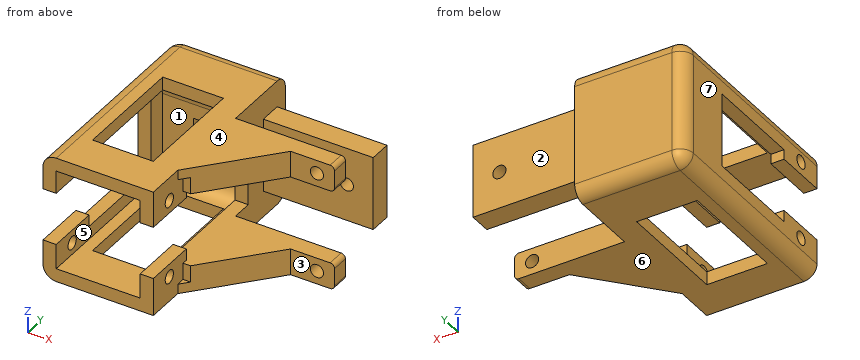
```python
from build123d import *

# Parameters (mm, degrees)
SKETCH4_W            = 25.1
SKETCH4_H            = 28.75
BOSS_EXTRUDE2_DEPTH  = 53
SKETCH5_W            = 19.1
SKETCH5_H            = 22.75
CUT_EXTRUDE1_DEPTH   = 21.67
FILLET1_R            = 4.1
SKETCH6_W            = 5
SKETCH6_H            = 8
CUT_EXTRUDE2_DEPTH   = 4.67
SKETCH7_W            = 16.769550268
SKETCH7_H            = 35.14
CUT_EXTRUDE3_DEPTH   = 40
SKETCH8_W            = 13.798322684
SKETCH8_H            = 35.14
CUT_EXTRUDE4_DEPTH   = 40
BOSS_EXTRUDE3_DEPTH  = 17
SKETCH10_W           = 3
SKETCH10_H           = 9
BOSS_EXTRUDE4_DEPTH  = 13.8
SKETCH11_W           = 3
SKETCH11_H           = 9
BOSS_EXTRUDE5_DEPTH  = 13.8
SKETCH12_W           = 3
SKETCH12_H           = 12
BOSS_EXTRUDE6_DEPTH  = 16.77
SKETCH24_R           = 1.5
CUT_EXTRUDE6_DEPTH   = 40.8
SKETCH25_W           = 28.75
SKETCH25_H           = 21.925089144
CUT_EXTRUDE7_DEPTH   = 40.8
SKETCH26_W           = 11.913987102
SKETCH26_H           = 12
CUT_EXTRUDE8_DEPTH   = 40.8
SKETCH30_W           = 28.75
SKETCH30_H           = 8.02
BOSS_EXTRUDE10_DEPTH = 30
SKETCH32_W           = 5.990224866
SKETCH32_H           = 21.060252184
BOSS_EXTRUDE13_DEPTH = 30
CUT_EXTRUDE9_DEPTH   = 30
SKETCH36_W           = 5
SKETCH36_H           = 28.75
CUT_EXTRUDE10_DEPTH  = 30
SKETCH38_W           = 5.99
SKETCH38_H           = 8.02
CUT_EXTRUDE11_DEPTH  = 25
SKETCH39_R           = 1.5
CUT_EXTRUDE12_DEPTH  = 25
SKETCH40_R           = 1.5
CUT_EXTRUDE13_DEPTH  = 25
FILLET4_R            = 3
FILLET5_R            = 3
FILLET7_R            = 1
SKETCH41_W           = 16.77
SKETCH41_H           = 3
CUT_EXTRUDE14_DEPTH  = 25
CUT_EXTRUDE15_DEPTH  = 3.79
CUT_EXTRUDE16_DEPTH  = 3.79


with BuildPart() as part:
    # Sketch4 → Boss-Extrude2 (new body)
    with BuildSketch(Plane(origin=(0, 0, 0), x_dir=(1, 0, 0), z_dir=(0, 1, 0))):
        Rectangle(SKETCH4_W, SKETCH4_H)
    extrude(amount=BOSS_EXTRUDE2_DEPTH)

    # Sketch5 → Cut-Extrude1 (cut)
    with BuildSketch(Plane(origin=(0, 0, 0), x_dir=(-1, 0, 0), z_dir=(0, -1, 0))):
        Rectangle(SKETCH5_W, SKETCH5_H)
    extrude(amount=-CUT_EXTRUDE1_DEPTH, mode=Mode.SUBTRACT)

    # Fillet1
    fillet1_edges = [part.edges().sort_by_distance(p)[0] for p in [
        (0, 21.67, -11.375),
        (0, 21.67, 11.375),
    ]]
    fillet(fillet1_edges, radius=FILLET1_R)

    # Sketch6 → Cut-Extrude2 (cut)
    with BuildSketch(Plane(origin=(0, 21.67, 0), x_dir=(-1, 0, 0), z_dir=(0, -1, 0))):
        Rectangle(SKETCH6_W, SKETCH6_H)
    extrude(amount=-CUT_EXTRUDE2_DEPTH, mode=Mode.SUBTRACT)

    # Sketch7 → Cut-Extrude3 (cut)
    with BuildSketch(Plane(origin=(12.55, 0, 0), x_dir=(0, 0, -1), z_dir=(1, 0, 0))):
        Rectangle(SKETCH7_W, SKETCH7_H)
    extrude(amount=-CUT_EXTRUDE3_DEPTH, mode=Mode.SUBTRACT)

    # Sketch8 → Cut-Extrude4 (cut)
    with BuildSketch(Plane(origin=(0, 0, -14.375), x_dir=(-1, 0, 0), z_dir=(0, 0, -1))):
        Rectangle(SKETCH8_W, SKETCH8_H)
    extrude(amount=-CUT_EXTRUDE4_DEPTH, mode=Mode.SUBTRACT)

    # Sketch9 → Boss-Extrude3 (add)
    with BuildSketch(Plane.XZ):
        Polygon((-9.55, 8.384775134), (-12.55, 8.384775134), (-12.55, 14.375), (-6.899161342, 14.375), (-6.899161342, 11.375), (-9.55, 11.375), align=None)
        Polygon((-9.55, -8.384775134), (-12.55, -8.384775134), (-12.55, -14.375), (-6.899161342, -14.375), (-6.899161342, -11.375), (-9.55, -11.375), align=None)
        Polygon((6.899161342, -11.375), (6.899161342, -14.375), (12.55, -14.375), (12.55, -8.384775134), (9.55, -8.384775134), (9.55, -11.375), align=None)
        Polygon((9.55, 8.384775134), (12.55, 8.384775134), (12.55, 14.375), (6.899161342, 14.375), (6.899161342, 11.375), (9.55, 11.375), align=None)
    extrude(amount=BOSS_EXTRUDE3_DEPTH)

    # Sketch10 → Boss-Extrude4 (add)
    with BuildSketch(Plane(origin=(-6.899161342, 0, 0), x_dir=(0, 0, -1), z_dir=(1, 0, 0))):
        with Locations((-12.875, -12.5)):
            Rectangle(SKETCH10_W, SKETCH10_H)
    extrude(amount=BOSS_EXTRUDE4_DEPTH)

    # Sketch11 → Boss-Extrude5 (add)
    with BuildSketch(Plane.ZY.offset(-6.899161342)):
        with Locations((-12.875, -12.5)):
            Rectangle(SKETCH11_W, SKETCH11_H)
    extrude(amount=BOSS_EXTRUDE5_DEPTH)

    # Sketch12 → Boss-Extrude6 (add)
    with BuildSketch(Plane.XY.offset(-8.384775134)):
        with Locations((-11.05, -11)):
            Rectangle(SKETCH12_W, SKETCH12_H)
        with Locations((11.05, -11)):
            Rectangle(SKETCH12_W, SKETCH12_H)
    extrude(amount=BOSS_EXTRUDE6_DEPTH)

    # Sketch24 → Cut-Extrude6 (cut)
    with BuildSketch(Plane(origin=(12.55, 0, 0), x_dir=(0, 0, -1), z_dir=(1, 0, 0))):
        with Locations((8.675, -11.18)):
            Circle(SKETCH24_R)
        with Locations((-9.075, -11.18)):
            Circle(SKETCH24_R)
    extrude(amount=-CUT_EXTRUDE6_DEPTH, mode=Mode.SUBTRACT)

    # Sketch25 → Cut-Extrude7 (cut)
    with BuildSketch(Plane.ZY.offset(12.55)):
        with Locations((0, 42.037455428)):
            Rectangle(SKETCH25_W, SKETCH25_H)
    extrude(amount=-CUT_EXTRUDE7_DEPTH, mode=Mode.SUBTRACT)

    # Sketch26 → Cut-Extrude8 (cut)
    with BuildSketch(Plane.ZY.offset(12.55)):
        with Locations((0.21531302, -11)):
            Rectangle(SKETCH26_W, SKETCH26_H)
    extrude(amount=-CUT_EXTRUDE8_DEPTH, mode=Mode.SUBTRACT)

    # Sketch30 → Boss-Extrude10 (add)
    with BuildSketch(Plane(origin=(12.55, 0, 0), x_dir=(0, 0, -1), z_dir=(1, 0, 0))):
        with Locations((0, 27.064910856)):
            Rectangle(SKETCH30_W, SKETCH30_H)
    extrude(amount=BOSS_EXTRUDE10_DEPTH)

    # Sketch32 → Boss-Extrude13 (add)
    with BuildSketch(Plane(origin=(12.55, 0, 0), x_dir=(0, 0, -1), z_dir=(1, 0, 0))):
        with Locations((-11.379887567, 2.424784764)):
            Rectangle(SKETCH32_W, SKETCH32_H)
        with Locations((11.379887567, 2.424784764)):
            Rectangle(SKETCH32_W, SKETCH32_H)
    extrude(amount=BOSS_EXTRUDE13_DEPTH)

    # Sketch35 → Cut-Extrude9 (cut)
    with BuildSketch(Plane(origin=(0, 0, -14.375), x_dir=(-1, 0, 0), z_dir=(0, 0, -1))):
        Polygon((-42.55, 8.954910856), (-27.55, 8.954910856), (-12.55, -8.105341328), (-42.55, -8.105341328), align=None)
    extrude(amount=-CUT_EXTRUDE9_DEPTH, mode=Mode.SUBTRACT)

    # Sketch36 → Cut-Extrude10 (cut)
    with BuildSketch(Plane(origin=(0, 31.074910856, 0), x_dir=(1, 0, 0), z_dir=(0, 1, 0))):
        with Locations((40.05, 0)):
            Rectangle(SKETCH36_W, SKETCH36_H)
    extrude(amount=-CUT_EXTRUDE10_DEPTH, mode=Mode.SUBTRACT)

    # Sketch38 → Cut-Extrude11 (cut)
    with BuildSketch(Plane(origin=(37.55, 0, 0), x_dir=(0, 0, -1), z_dir=(1, 0, 0))):
        with Locations((-11.38, 27.064910856)):
            Rectangle(SKETCH38_W, SKETCH38_H)
        with Locations((11.38, 27.064910856)):
            Rectangle(SKETCH38_W, SKETCH38_H)
    extrude(amount=-CUT_EXTRUDE11_DEPTH, mode=Mode.SUBTRACT)

    # Sketch39 → Cut-Extrude12 (cut)
    with BuildSketch(Plane(origin=(0, 8.954910856, 0), x_dir=(-1, 0, 0), z_dir=(0, -1, 0))):
        with Locations(Location((-33.55, 11.379887567, 0), (0, 0, 90))):
            Circle(SKETCH39_R)
        with Locations(Location((-33.55, -11.379887567, 0), (0, 0, 90))):
            Circle(SKETCH39_R)
    extrude(amount=-CUT_EXTRUDE12_DEPTH, mode=Mode.SUBTRACT)

    # Sketch40 → Cut-Extrude13 (cut)
    with BuildSketch(Plane.XZ.offset(-23.054910856)):
        with Locations(Location((31.55, 0, 0), (0, 0, 270))):
            Circle(SKETCH40_R)
    extrude(amount=-CUT_EXTRUDE13_DEPTH, mode=Mode.SUBTRACT)

    # Fillet4
    fillet4_edges = [part.edges().sort_by_distance(p)[0] for p in [
        (-12.55, 31.074910856, 0),
        (0, 31.074910856, 14.375),
        (0, 31.074910856, -14.375),
    ]]
    fillet(fillet4_edges, radius=FILLET4_R)

    # Fillet5
    # the kernel refuses this fillet: 3 mm, written as the material it takes off along each edge
    with BuildSketch(Plane(origin=(-9.55, 28.074910856, 11.375), x_dir=(0, 0, 1), z_dir=(-1, 0, 0))) as fillet5_piece_1_section:
        Polygon((0, 0), (FILLET5_R, 0), (FILLET5_R, FILLET5_R), (0, FILLET5_R), align=None)
    fillet5_piece_1 = extrude(amount=FILLET5_R, mode=Mode.PRIVATE)
    fillet5_piece_1 = fillet5_piece_1 - Plane(origin=(-9.55, 28.074910856, 11.375), x_dir=(0, -0.7071067811865475, -0.7071067811865475), z_dir=(-1, 0, 0)) * Sphere(FILLET5_R, mode=Mode.PRIVATE)
    add(fillet5_piece_1, mode=Mode.SUBTRACT)
    with BuildSketch(Plane(origin=(-9.55, 28.074910856, -11.375), x_dir=(-1, 0, 0), z_dir=(0, 0, -1))) as fillet5_piece_2_section:
        Polygon((0, 0), (FILLET5_R, 0), (FILLET5_R, FILLET5_R), (0, FILLET5_R), align=None)
    fillet5_piece_2 = extrude(amount=FILLET5_R, mode=Mode.PRIVATE)
    fillet5_piece_2 = fillet5_piece_2 - Plane(origin=(-9.55, 28.074910856, -11.375), x_dir=(0.7071067811865475, -0.7071067811865475, 0), z_dir=(0, 0, -1)) * Sphere(FILLET5_R, mode=Mode.PRIVATE)
    add(fillet5_piece_2, mode=Mode.SUBTRACT)
    with BuildSketch(Plane(origin=(-12.55, 28.074910856, -14.375), x_dir=(1, 0, 0), z_dir=(0, -1, 0))) as fillet5_piece_3:
        with BuildLine():
            CenterArc((FILLET5_R, FILLET5_R), FILLET5_R, 180, 90)
            Line((0, FILLET5_R), (0, 0))
            Line((0, 0), (FILLET5_R, 0))
        make_face()
    extrude(amount=52.574910856, mode=Mode.SUBTRACT)
    with BuildSketch(Plane(origin=(-12.55, -24.5, 14.375), x_dir=(0, 0, -1), z_dir=(0, 1, 0))) as fillet5_piece_4:
        with BuildLine():
            CenterArc((FILLET5_R, -FILLET5_R), FILLET5_R, 90, 90)
            Line((0, -FILLET5_R), (0, 0))
            Line((0, 0), (FILLET5_R, 0))
        make_face()
    extrude(amount=52.574910856, mode=Mode.SUBTRACT)

    # Fillet7
    fillet7_edges = [part.edges().sort_by_distance(p)[0] for p in [
        (37.55, 10.954910856, -14.375),
        (37.55, 10.954910856, -8.384775134),
        (37.55, 10.954910856, 14.375),
        (37.55, 10.954910856, 8.384775134),
    ]]
    fillet(fillet7_edges, radius=FILLET7_R)

    # Sketch41 → Cut-Extrude14 (cut)
    with BuildSketch(Plane(origin=(37.55, 0, 0), x_dir=(0, 0, -1), z_dir=(1, 0, 0))):
        with Locations((0, 29.574910856)):
            Rectangle(SKETCH41_W, SKETCH41_H)
    extrude(amount=-CUT_EXTRUDE14_DEPTH, mode=Mode.SUBTRACT)

    # Sketch43 → Cut-Extrude15 (cut)
    with BuildSketch(Plane(origin=(0, 0, 8.384775134), x_dir=(-1, 0, 0), z_dir=(0, 0, -1))):
        Polygon((-12.55, -8.105341328), (-12.55, -6.175341328), (-14.24692685, -6.175341328), align=None)
    extrude(amount=-CUT_EXTRUDE15_DEPTH, mode=Mode.SUBTRACT)

    # Sketch44 → Cut-Extrude16 (cut)
    with BuildSketch(Plane.XY.offset(-8.384775134)):
        Polygon((12.55, -8.105341328), (12.55, -6.175341328), (14.24692685, -6.175341328), align=None)
    extrude(amount=-CUT_EXTRUDE16_DEPTH, mode=Mode.SUBTRACT)


solid = part.part
```
Can you work these out from the model? Positions are in its coordinate system, mm. Face numbers are marked on the shaded views. A direction names the side the tool comes from. Give positions to 0.01 mm unless a question says otherwise; leave off trailing zeros. Order: outer loops, then holes, each group sorted by start corner. A loop starts at its lowest first (then second) coordinate and runs counter-clockwise, first axis right, second up. Notation, with made-up numbers: M 62,52 L 111,52 A12 cw 111,73 Z; hole C 81.5,-1 d7. An arc over 180 degrees is marked long. One line per item, written item: value.
1) I want a section at C-C, the plane z = 0. List the corners of the cut face in (x, y) for me, plus the area to 3 significant figures.
Answer sheet:
outline: M -12.55,17.57 L -9.55,17.57 L -9.55,21.67 L -2.5,21.67 L -2.5,26.34 L 2.5,26.34 L 2.5,21.67 L 9.55,21.67 L 9.55,17.57 L 12.55,17.57 L 12.55,23.05 L 30.05,23.05 L 30.05,28.07 L 12.55,28.07 L 12.55,31.07 L -9.55,31.07 A3 ccw -12.55,28.07 Z; M 33.05,23.05 L 37.55,23.05 L 37.55,28.07 L 33.05,28.07 Z
area: 346 mm^2
2) For P1, Ø3, axis at x = 18.5, z = -4, coming from the +Y side; P2, Ø7.5, axis at x = 4.5, z = 2, coming from the -Y side; P3, Ø2.5, axis at y = 0.5, z = -13.5, coming from the +X side, each with a flat end and sliding along its axis, tell me the tip position at first contact or that it passes through.
Answer sheet:
P1: stops at y = 28.07
P2: stops at y = 21.67
P3: stops at x = 21.22
3) We'd pull the mould along Z, two halves only. Please class the marked faces 5, 6 and 7: released by +Z, released by -Z, zero draft, split by the parting line, or undercut.
Answer sheet:
face 5: undercut
face 6: released by -Z
face 7: zero draft
4) Please list where these lines run through material, in increasing order: line 1 along Z through (x, y) = (-8.5, 14.5) (3 decimals); line 2 along X through (y, z) = (17, -9.25); line 3 along Z through (x, y) = (20, 2) (3 decimals).
Answer sheet:
line 1: z = -14.375 to -11.375, 11.375 to 14.375
line 2: x = -12.55 to -9.55, 9.55 to 12.55
line 3: z = -14.375 to -8.385, 8.385 to 14.375
5) On a 3-axis mill with a long thin cutter (end or side, diameter ignored), from which of +Z, -Z, +X, -X, +Y, -Y can I reach the whole of each face in a straight line? I mean the marked faces 1, 2, 3 and 4. Say none if no direction works.
Answer sheet:
face 1: -Y
face 2: +Z, -Z, +X, +Y
face 3: +Z, -Z, +X, -Y
face 4: +Z, +X, -X, +Y, -Y
6) I want a section at B-B, the plane y = -11.18. Count the separate pieces of the cut face and the enclosed holes in it, plus the area to 3 significant figures.
Answer sheet:
separate pieces: 6
enclosed holes: 0
area: 176 mm^2
7) I want a section at A-A, the plane x = 1.5. List the corners of the cut face in (y, z) for me (3 decimals), plus the area to 3 significant figures.
Answer sheet:
outline: M -17,-14.375 L -8,-14.375 L -8,-11.375 L -17,-11.375 Z; M -17,11.375 L -8,11.375 L -8,14.375 L -17,14.375 Z; M 17.57,-14.375 L 28.075,-14.375 A3 ccw 31.075,-11.375 L 31.075,11.375 A3 ccw 28.075,14.375 L 17.57,14.375 L 17.57,11.375 A4.1 cw 21.67,7.275 L 21.67,4 L 26.34,4 L 26.34,-4 L 21.67,-4 L 21.67,-7.275 A4.1 cw 17.57,-11.375 Z
area: 315 mm^2
8) I want a section at D-D, the plane y = -1. List the corners of the cut face in (x, z) for me (3 decimals), plus the area to 3 significant figures.
Answer sheet:
outline: M -12.55,-11.375 A3 ccw -9.55,-14.375 L -6.899,-14.375 L -6.899,-11.375 L -9.55,-11.375 L -9.55,-8.385 L -12.55,-8.385 Z; M -12.55,8.385 L -9.55,8.385 L -9.55,11.375 L -6.899,11.375 L -6.899,14.375 L -9.55,14.375 A3 ccw -12.55,11.375 Z; M 6.899,-14.375 L 18.797,-14.375 L 18.797,-8.385 L 9.55,-8.385 L 9.55,-11.375 L 6.899,-11.375 Z; M 6.899,11.375 L 9.55,11.375 L 9.55,8.385 L 18.797,8.385 L 18.797,14.375 L 6.899,14.375 Z
area: 175 mm^2
